Autodesk Inventor part; units mm, degrees
ref_plane "YZ Plane" through (0, 0, 0) normal (1, 0, 0) x (0, 1, 0)
ref_plane "XZ Plane" through (0, 0, 0) normal (0, 1, 0) x (-1, 0, 0)
ref_plane "XY Plane" through (0, 0, 0) normal (0, 0, 1) x (1, 0, 0)
sketch "Sketch1" plane through (0, 0, 0) normal (0, 0, 1) x (1, 0, 0)
  circle A0 centre (0, 0) radius 6.35
  circle A1 centre (0, 0) radius 21.3337
  arc A2 (28.7594, 8.538) -> (28.7594, -8.538) centre (30, 0) ccw
  arc A3 (16.5428, 25.0267) -> (27.5191, 11.9457) centre (22.9813, 19.2836) ccw
  arc A4 (-3.4143, 29.8051) -> (13.4023, 26.8399) centre (5.2094, 29.5442) ccw
  arc A5 (-21.7738, 20.6373) -> (-6.9856, 29.1754) centre (-15, 25.9808) ccw
  arc A6 (-29.9452, 1.8132) -> (-24.1048, 17.8594) centre (-28.1908, 10.2606) ccw
  arc A7 (-24.1048, -17.8594) -> (-29.9452, -1.8132) centre (-28.1908, -10.2606) ccw
  arc A8 (-6.9856, -29.1754) -> (-21.7738, -20.6373) centre (-15, -25.9808) ccw
  arc A9 (13.4023, -26.8399) -> (-3.4143, -29.8051) centre (5.2094, -29.5442) ccw
  arc A10 (27.5191, -11.9457) -> (16.5428, -25.0267) centre (22.9813, -19.2836) ccw
  arc A11 (27.5191, -11.9457) -> (28.7594, -8.538) centre (0, 0) ccw
  arc A12 (28.7594, 8.538) -> (27.5191, 11.9457) centre (0, 0) ccw
  arc A13 (16.5428, 25.0267) -> (13.4023, 26.8399) centre (0, 0) ccw
  arc A14 (-3.4143, 29.8051) -> (-6.9856, 29.1754) centre (0, 0) ccw
  arc A15 (-21.7738, 20.6373) -> (-24.1048, 17.8594) centre (0, 0) ccw
  arc A16 (-29.9452, 1.8132) -> (-29.9452, -1.8132) centre (0, 0) ccw
  arc A17 (-24.1048, -17.8594) -> (-21.7738, -20.6373) centre (0, 0) ccw
  arc A18 (-6.9856, -29.1754) -> (-3.4143, -29.8051) centre (0, 0) ccw
  arc A19 (13.4023, -26.8399) -> (16.5428, -25.0267) centre (0, 0) ccw
  arc A20 (-6.3913, -25.4085) -> (-2.6843, -26.0621) centre (0, 0) ccw
  point P0 (25.2001, -7.1692)
  point P1 (25.2001, 7.1692)
  point P2 (23.9126, 10.7064)
  point P3 (14.6961, 21.6902)
  point P4 (11.4362, 23.5723)
  point P5 (-2.6843, 26.0621)
  point P6 (-6.3913, 25.4085)
  point P7 (-18.8087, 18.2393)
  point P8 (-21.2283, 15.3558)
  point P9 (-26.1323, 1.8821)
  point P10 (-26.1323, -1.8821)
  point P11 (-21.2283, -15.3558)
  point P12 (-18.8087, -18.2393)
  point P13 (11.4362, -23.5723)
  point P14 (23.9126, -10.7064)
  point P15 (14.6961, -21.6902)
  dimension "d1" = 12.7
  dimension "d5" = 360
extrude "Extrusion1" add sketch "Sketch1" along normal blind 5 contours A0 | A1 | A2 A11 A10 A19 A9 A20 A8 A17 A7 A16 A6 A15 A5 A14 A4 A13 A3 A12 | A9 A18 A8 A20
sketch "Sketch2" plane through (0, 0, 5) normal (0, 0, 1) x (1, 0, 0)
  circle A0 centre (0, 0) radius 6.35
  dimension "d9" = 12.7
extrude "Extrusion2" cut sketch "Sketch2" against normal through all
sketch "Sketch3" plane through (0, 0, 5) normal (0, 0, 1) x (1, 0, 0)
  circle A0 centre (0, 0) radius 12.5
  circle A1 centre (0, 0) radius 6.35
  dimension "d12" = 25
  dimension "d13" = 12.7
extrude "Extrusion3" add sketch "Sketch3" along normal blind 2
sketch "Sketch4" plane through (0, 0, 0) normal (0, 0, -1) x (-1, 0, 0)
  circle A0 centre (0, 0) radius 6.35
  circle A1 centre (0, 0) radius 12.5
  dimension "d16" = 12.7
  dimension "d17" = 25
extrude "Extrusion4" add sketch "Sketch4" along normal blind 2
properties part number "Gear"
The listing builds one solid part. Answer for the finished solid, in the listing's coordinates (mm). A direction names the side the tool comes from. Give positions to 0.01 mm unless a question says otherwise; leave off trailing zeros. Loops run counter-clockwise (first coordinate to the right, second up) from the corner with the lowest first, then second, coordinate; pieces in that order, holes last. Notation, with made-up numbers: M 30.5,69 L 77.5,69 A20 ccw 77.5,89 Z; hole C 4,-18 d1. An arc over 180 degrees is marked long. One line per item, written item: value.
1. For a pull along Y with two mould halves and no side action, classify faces 1 (the face through (16.263, -13.871, 2.465)), 2 (the face through (-6, 3, 7)), 3 (the face through (28.2, -10.24, 2.46)) as pulls with the +Y half, pulls with the -Y half, needs draft (parallel to the pull), parting line crosses it, or undercut.
Found:
face 1: undercut
face 2: needs draft
face 3: pulls with the -Y half
2. For faces 4 (the face through (21.374, -0.172, 2.465)), 5 (the face through (-1, -13, 5)), determine the directions among +Z, -Z, +X, -X, +Y, -Y from which every point of the face is accessible in a straight line to the end or side of a thin tool.
Found:
face 4: +Z, -Z, +X
face 5: +Z
3. Find the intervals of material crossed by probe 1 along X at (y, z) = (0, 3.65); probe 2 along Y at (x, z) = (0, -1.25); probe 3 along Y at (x, z) = (0, 1.15), in increasing order.
Found:
probe 1: -30 to -6.35, 6.35 to 21.37
probe 2: -12.5 to -6.35, 6.35 to 12.5
probe 3: -22.67 to -6.35, 6.35 to 22.67
4. Section C-C on x = 0 is taken. Determine the outline of the cut face in (y, z), plus the area to 3 significant figures.
Found:
outline: M -22.67,0 L -12.5,0 L -12.5,-2 L -6.35,-2 L -6.35,7 L -12.5,7 L -12.5,5 L -22.67,5 Z; M 6.35,-2 L 12.5,-2 L 12.5,0 L 22.67,0 L 22.67,5 L 12.5,5 L 12.5,7 L 6.35,7 Z
area: 212 mm^2
5. Each of these flat-tipped pins is pushed along its axis until it touches: P1, Ø5, axis at y = -18.5, z = 5.5, coming from the +X side; P2, Ø3, axis at y = -9, z = 2.5, coming from the -X side; P3, Ø4, axis at y = -8, z = 2.5, coming from the +X side. Where does it stop, or does it pass through?
Found:
P1: x = 14.98
P2: x = -20.02
P3: x = 28.76
6. Section B-B on y = 0 is taken. Determine the outline of the cut face in (x, z), plus the area to 3 significant figures.
Found:
outline: M -30,0 L -12.5,0 L -12.5,-2 L -6.35,-2 L -6.35,7 L -12.5,7 L -12.5,5 L -30,5 Z; M 6.35,-2 L 12.5,-2 L 12.5,0 L 21.37,0 L 21.37,5 L 12.5,5 L 12.5,7 L 6.35,7 Z
area: 243 mm^2
7. Section A-A on z = 1.75 is taken. Determine the outline of the cut face in (x, y).
Found:
outline: M -29.95,-1.81 A8.63 cw -24.1,-17.86 A29.99 ccw -21.77,-20.64 A8.63 cw -6.99,-29.18 A29.99 ccw -3.41,-29.81 A8.63 cw 13.4,-26.84 A29.99 ccw 16.54,-25.03 A8.63 cw 27.52,-11.95 A30 ccw 28.76,-8.54 A8.63 cw 28.76,8.54 A30 ccw 27.52,11.95 A8.63 cw 16.54,25.03 A30.01 ccw 13.4,26.84 A8.63 cw -3.41,29.81 A30.01 ccw -6.99,29.18 A8.63 cw -21.77,20.64 A30.01 ccw -24.1,17.86 A8.63 cw -29.95,1.81 A30 ccw Z; hole C 0,0 d12.7
8. Section D-D on y = -7.5 is taken. Determine the outline of the cut face in (x, z).
Found:
outline: M -20.02,0 L -10,0 L -10,-2 L 10,-2 L 10,0 L 25.74,0 L 25.74,5 L 10,5 L 10,7 L -10,7 L -10,5 L -20.02,5 Z
